from build123d import *

# Parameters (mm, degrees)
SKETCH_1_W            = 40.4
SKETCH_1_H            = 21.6
EXTRUDE_1_DEPTH       = 19.8
SKETCH_3_W            = 38.4
SKETCH_3_H            = 17.9
EXTRUDE_2_DEPTH       = 1
SKETCH_4_W            = 40.4
SKETCH_4_H            = 19.8
EXTRUDE_3_DEPTH       = 0.5
SKETCH_5_R            = 2.75
EXTRUDE_4_DEPTH       = 0.5
EXTRUDE_5_DEPTH       = 0.8
SKETCH_7_R            = 3
EXTRUDE_6_DEPTH       = 2.1
SKETCH_8_R            = 1.9
CUT_EXTRUDE_7_DEPTH   = 38.750231787
SKETCH_10_R           = 0.75
CUT_EXTRUDE_10_DEPTH  = 2.7
EXTRUDE_11_DEPTH      = 1.3
SKETCH_13_R           = 3
CUT_EXTRUDE_13_DEPTH  = 37.710216562
EXTRUDE_START         = -1.3
EXTRUDE_14_DEPTH      = 4.6
SKETCH_14_R           = 2
CUT_EXTRUDE_15_DEPTH  = 39.896915045
EXTRUDE_16_DEPTH      = 0.5
EXTRUDE_16_DEPTH_BACK = 2
SKETCH_15_R           = 2
SKETCH_16_R           = 0.75
CUT_EXTRUDE_17_DEPTH  = 2.3
SKETCH_17_W           = 38.6
SKETCH_17_H           = 18
CUT_EXTRUDE_18_DEPTH  = 20
EXTRUDE_START_2       = 18
SKETCH_18_W           = 38.6
SKETCH_18_H           = 18
EXTRUDE_19_DEPTH      = 18
SKETCH_19_R           = 0.8
CUT_EXTRUDE_20_DEPTH  = 27.4
SKETCH_20_R           = 8.6
CUT_EXTRUDE_21_DEPTH  = 27.4
SKETCH_21_R           = 1.05
EXTRUDE_22_DEPTH      = 0.5
SKETCH_22_R           = 0.75
CUT_EXTRUDE_23_DEPTH  = 0.1
CUT_EXTRUDE_24_REACH  = 37.896
SKETCH_23_R           = 0.5
CUT_EXTRUDE_27_REACH  = 49.887
SKETCH_25_R           = 2
SKETCH_25_W           = 5
SKETCH_25_H           = 1


with BuildPart() as part:
    # 草圖1 → 伸長1 (new body)
    with BuildSketch(Plane.XY):
        Rectangle(SKETCH_1_W, SKETCH_1_H)
    extrude(amount=EXTRUDE_1_DEPTH)

    # 草圖3 → 伸長2 (add)
    with BuildSketch(Plane(origin=(0, 10.8, 0), x_dir=(1, 0, 0), z_dir=(0, 1, 0))):
        with Locations((0, -9.9)):
            Rectangle(SKETCH_3_W, SKETCH_3_H)
        with BuildLine():
            Line((-15.485164876, -1.75), (15.485164876, -1.75))
            ThreePointArc((15.485164876, -1.75), (16.512994231, -3.637005769), (18.4, -4.664835124))
            Line((18.4, -4.664835124), (18.4, -15.135164876))
            ThreePointArc((18.4, -15.135164876), (16.512994231, -16.162994231), (15.485164876, -18.05))
            Line((15.485164876, -18.05), (-15.485164876, -18.05))
            ThreePointArc((-15.485164876, -18.05), (-16.512994231, -16.162994231), (-18.4, -15.135164876))
            Line((-18.4, -15.135164876), (-18.4, -4.664835124))
            ThreePointArc((-18.4, -4.664835124), (-16.512994231, -3.637005769), (-15.485164876, -1.75))
        make_face(mode=Mode.SUBTRACT)
    extrude(amount=EXTRUDE_2_DEPTH)

    # 草圖4 → 伸長3 (add)
    with BuildSketch(Plane(origin=(0, 10.8, 0), x_dir=(1, 0, 0), z_dir=(0, 1, 0))):
        with Locations((0, -9.9)):
            Rectangle(SKETCH_4_W, SKETCH_4_H)
    extrude(amount=EXTRUDE_3_DEPTH)

    # 草圖5 → 伸長4 (add)
    with BuildSketch(Plane(origin=(0, 11.3, 0), x_dir=(1, 0, 0), z_dir=(0, 1, 0))):
        with Locations(Location((-1.55, -9.9, 0), (0, 0, 270))):
            Circle(SKETCH_5_R)
    extrude(amount=EXTRUDE_4_DEPTH)

    # 草圖6 → 伸長5 (add)
    with BuildSketch(Plane(origin=(0, 11.3, 0), x_dir=(1, 0, 0), z_dir=(0, 1, 0))):
        with BuildLine():
            Line((6.2, -7.31930242), (6.2, -12.48069758))
            ThreePointArc((6.2, -12.48069758), (13.6, -9.9), (6.2, -7.31930242))
        make_face()
    extrude(amount=EXTRUDE_5_DEPTH)

    # 草圖7 → 伸長6 (add)
    with BuildSketch(Plane(origin=(0, 12.1, 0), x_dir=(1, 0, 0), z_dir=(0, 1, 0))):
        with Locations(Location((9.45, -9.9, 0), (0, 0, 270))):
            Circle(SKETCH_7_R)
    extrude(amount=EXTRUDE_6_DEPTH)

    # 草圖8 → 伸長7 (cut, through all)
    with BuildSketch(Plane(origin=(0, 14.2, 0), x_dir=(1, 0, 0), z_dir=(0, 1, 0))):
        with Locations(Location((9.45, -9.9, 0), (0, 0, 270))):
            Circle(SKETCH_8_R)
    extrude(amount=-CUT_EXTRUDE_7_DEPTH, mode=Mode.SUBTRACT)

    # 草圖10 → 伸長10 (cut)
    with BuildSketch(Plane(origin=(0, 11.8, 0), x_dir=(1, 0, 0), z_dir=(0, 1, 0))):
        with Locations(Location((-1.55, -9.9, 0), (0, 0, 270))):
            Circle(SKETCH_10_R)
    extrude(amount=-CUT_EXTRUDE_10_DEPTH, mode=Mode.SUBTRACT)

    # 草圖11 → 伸長11 (add)
    with BuildSketch(Plane(origin=(0, 11.3, 0), x_dir=(1, 0, 0), z_dir=(0, 1, 0))):
        with BuildLine():
            Line((-11.95, -5.837980798), (-11.95, -13.962019202))
            ThreePointArc((-11.95, -13.962019202), (-14.95, -9.9), (-11.95, -5.837980798))
        make_face()
    extrude(amount=EXTRUDE_11_DEPTH)

    # 草圖13 → 伸長13 (cut, through all)
    with BuildSketch(Plane(origin=(0, 12.6, 0), x_dir=(1, 0, 0), z_dir=(0, 1, 0))):
        with Locations(Location((-10.7, -9.9, 0), (0, 0, 270))):
            Circle(SKETCH_13_R)
    extrude(amount=-CUT_EXTRUDE_13_DEPTH, mode=Mode.SUBTRACT)

    # 草圖12 → 伸長14 (add)
    with BuildSketch(Plane(origin=(0, 12.6, 0), x_dir=(1, 0, 0), z_dir=(0, 1, 0)).offset(EXTRUDE_START)):
        with BuildLine():
            Line((-9.420351611, -6.75), (-9.420351611, -13.05))
            ThreePointArc((-9.420351611, -13.05), (-14.1, -9.9), (-9.420351611, -6.75))
        make_face()
    extrude(amount=EXTRUDE_14_DEPTH)

    # 草圖14 → 伸長15 (cut, through all)
    with BuildSketch(Plane(origin=(0, 15.9, 0), x_dir=(1, 0, 0), z_dir=(0, 1, 0))):
        with Locations((-10.7, -9.9)):
            Circle(SKETCH_14_R)
    extrude(amount=-CUT_EXTRUDE_15_DEPTH, mode=Mode.SUBTRACT)

    # 草圖15 → 伸長16 (add, two sides: drawn at the far end of the back side and taken through both)
    with BuildSketch(Plane(origin=(0, 15.9, 0), x_dir=(1, 0, 0), z_dir=(0, 1, 0)).offset(-EXTRUDE_16_DEPTH_BACK)):
        with Locations(Location((-10.7, -9.9, 0), (0, 0, 270))):
            Circle(SKETCH_15_R)
    extrude(amount=EXTRUDE_16_DEPTH + EXTRUDE_16_DEPTH_BACK)

    # 草圖16 → 伸長17 (cut)
    with BuildSketch(Plane(origin=(0, 16.4, 0), x_dir=(1, 0, 0), z_dir=(0, 1, 0))):
        with Locations(Location((-10.7, -9.9, 0), (0, 0, 270))):
            Circle(SKETCH_16_R)
    extrude(amount=-CUT_EXTRUDE_17_DEPTH, mode=Mode.SUBTRACT)

    # 草圖17 → 伸長18 (cut)
    with BuildSketch(Plane.XZ.offset(10.8)):
        with Locations((0, 9.9)):
            Rectangle(SKETCH_17_W, SKETCH_17_H)
    extrude(amount=-CUT_EXTRUDE_18_DEPTH, mode=Mode.SUBTRACT)

    # 草圖18 → 伸長19 (add)
    with BuildSketch(Plane.XZ.offset(-9.2).offset(EXTRUDE_START_2)):
        with Locations((0, 9.9)):
            Rectangle(SKETCH_18_W, SKETCH_18_H)
        with BuildLine():
            Line((15.485164876, 1.75), (-15.485164876, 1.75))
            ThreePointArc((-15.485164876, 1.75), (-16.512994231, 3.637005769), (-18.4, 4.664835124))
            Line((-18.4, 4.664835124), (-18.4, 15.135164876))
            ThreePointArc((-18.4, 15.135164876), (-16.512994231, 16.162994231), (-15.485164876, 18.05))
            Line((-15.485164876, 18.05), (15.485164876, 18.05))
            ThreePointArc((15.485164876, 18.05), (16.512994231, 16.162994231), (18.4, 15.135164876))
            Line((18.4, 15.135164876), (18.4, 4.664835124))
            ThreePointArc((18.4, 4.664835124), (16.512994231, 3.637005769), (15.485164876, 1.75))
        make_face(mode=Mode.SUBTRACT)
    extrude(amount=-EXTRUDE_19_DEPTH)

    # 草圖19 → 伸長20 (cut)
    with BuildSketch(Plane(origin=(0, 11.8, 0), x_dir=(1, 0, 0), z_dir=(0, 1, 0))):
        with Locations(Location((-17.7, -2.5, 0), (0, 0, 270))):
            Circle(SKETCH_19_R)
        with Locations(Location((17.7, -2.5, 0), (0, 0, 270))):
            Circle(SKETCH_19_R)
        with Locations(Location((17.7, -17.3, 0), (0, 0, 270))):
            Circle(SKETCH_19_R)
        with Locations(Location((-17.7, -17.3, 0), (0, 0, 270))):
            Circle(SKETCH_19_R)
    extrude(amount=-CUT_EXTRUDE_20_DEPTH, mode=Mode.SUBTRACT)

    # 草圖20 → 伸長21 (cut)
    with BuildSketch(Plane.XZ.offset(-9.2)):
        with Locations((-10.7, 9.9)):
            Circle(SKETCH_20_R)
    extrude(amount=CUT_EXTRUDE_21_DEPTH, mode=Mode.SUBTRACT)

    # 草圖21 → 伸長22 (add)
    with BuildSketch(Plane.XZ.offset(-9.2)):
        with Locations(Location((-1.55, 9.9, 0), (0, 0, 270))):
            Circle(SKETCH_21_R)
    extrude(amount=EXTRUDE_22_DEPTH)

    # 草圖22 → 伸長23 (cut)
    with BuildSketch(Plane(origin=(0, 9.2, 0), x_dir=(1, 0, 0), z_dir=(0, 1, 0))):
        with Locations(Location((-1.55, -9.9, 0), (0, 0, 270))):
            Circle(SKETCH_22_R)
    extrude(amount=-CUT_EXTRUDE_23_DEPTH, mode=Mode.SUBTRACT)

    # 草圖23 → 伸長24 (cut, up to next)
    with BuildSketch(Plane(origin=(0, 11.3, 0), x_dir=(1, 0, 0), z_dir=(0, 1, 0)), mode=Mode.PRIVATE) as cut_extrude_24_sk1:
        with Locations(Location((-10.7, -4.15, 0), (0, 0, 270))):
            Circle(SKETCH_23_R)
    cut_extrude_24_tool1 = extrude(cut_extrude_24_sk1.sketch, amount=-CUT_EXTRUDE_24_REACH, mode=Mode.PRIVATE) & part.part
    # 草圖23 → 伸長24 (cut, up to next)
    with BuildSketch(Plane(origin=(0, 11.3, 0), x_dir=(1, 0, 0), z_dir=(0, 1, 0)), mode=Mode.PRIVATE) as cut_extrude_24_sk2:
        with Locations(Location((-10.7, -15.65, 0), (0, 0, 270))):
            Circle(SKETCH_23_R)
    cut_extrude_24_tool2 = extrude(cut_extrude_24_sk2.sketch, amount=-CUT_EXTRUDE_24_REACH, mode=Mode.PRIVATE) & part.part
    add(cut_extrude_24_tool1.solids().sort_by_distance((-10.7, 11.3, 4.15))[0], mode=Mode.SUBTRACT)
    add(cut_extrude_24_tool2.solids().sort_by_distance((-10.7, 11.3, 15.65))[0], mode=Mode.SUBTRACT)

    # 伸長27: up to this face of the body (flat: up to its plane)
    cut_extrude_27_end = Plane(part.part.faces().sort_by_distance((18.4, 0.2, 9.9))[0])
    # 草圖25 → 伸長27 (cut, up to the picked face)
    with BuildSketch(Plane(origin=(20.2, 0, 0), x_dir=(0, 0, -1), z_dir=(1, 0, 0)), mode=Mode.PRIVATE) as cut_extrude_27_sk1:
        with Locations(Location((-9.9, -3.2, 0), (0, 0, 90))):
            Circle(SKETCH_25_R)
    cut_extrude_27_tool1 = split(extrude(cut_extrude_27_sk1.sketch, amount=-CUT_EXTRUDE_27_REACH, mode=Mode.PRIVATE), bisect_by=cut_extrude_27_end, keep=Keep.BOTH, mode=Mode.PRIVATE)
    # 草圖25 → 伸長27 (cut, up to the picked face)
    with BuildSketch(Plane(origin=(20.2, 0, 0), x_dir=(0, 0, -1), z_dir=(1, 0, 0)), mode=Mode.PRIVATE) as cut_extrude_27_sk2:
        with Locations((-9.9, -10.3)):
            Rectangle(SKETCH_25_W, SKETCH_25_H)
    cut_extrude_27_tool2 = split(extrude(cut_extrude_27_sk2.sketch, amount=-CUT_EXTRUDE_27_REACH, mode=Mode.PRIVATE), bisect_by=cut_extrude_27_end, keep=Keep.BOTH, mode=Mode.PRIVATE)
    add(cut_extrude_27_tool1.solids().sort_by(Axis((20.2, -3.2, 9.9), (-1, 0, 0)))[0], mode=Mode.SUBTRACT)
    add(cut_extrude_27_tool2.solids().sort_by(Axis((20.2, -10.3, 9.9), (-1, 0, 0)))[0], mode=Mode.SUBTRACT)


solid = part.part
For this review, take the finished solid that the model builds, in its own axes (mm). A direction names the side the tool comes from. Give positions to 0.01 mm unless a question says otherwise; leave off trailing zeros. Order: outer loops, then holes, each group sorted by start corner. A loop starts at its lowest first (then second) coordinate and runs counter-clockwise, first axis right, second up. Notation, with made-up numbers: (-36, 81.5) -> (15, 81.5) arc R15 ccw to (15, 109.5) -> close; hole circle Ø1 at (15.25, 32.5). An arc over 180 degrees is marked (long way). Write item = value, one per line.
1) To check wall thickness, follow L1, parallel to Z at x = -10.5, y = 6; L2, parallel to Z at x = -11.5, y = -9.25; L3, parallel to X at y = -9, z = 14.5. State the ranges of each line that lie inside material, in increasing order. Write a range as from..to.
Findings:
L1 = 0..1.3, 18.5..19.8
L2 = 0..0.9, 18.9..19.8
L3 = -20.2..-19.3, 19.3..20.2
2) Insertion check: pin 1 (2.5 mm diameter, centred on x = 17.7, z = 2.5, fed in from -Y); pin 2 (0.6 mm diameter, centred on x = -6.5, y = 11.5, fed in from +Z); pin 3 (6 mm diameter, centred on x = -1.5, z = 8, fed in from +Y); pin 4 (0.6 mm diameter, centred on x = -1, z = 10, fed in from -Y). Each pin has a flat end and moves straight along its axis. Give the tip position at first contact, or say it passes through.
Findings:
pin_1 = -8.8
pin_2 = 19.8
pin_3 = 11.8
pin_4 = 8.7
3) We need section B-B, the plane y = 10.25. Count the separate pieces of the cut face and the enclosed holes in it, and give its area (3 significant figures).
Findings:
separate_pieces = 1
enclosed_holes = 9
area = 749 mm^2
4) We need section C-C, the plane y = 4.75. Give the boundary of the cut face in (x, z).
Findings:
outline = (-20.2, 0) -> (20.2, 0) -> (20.2, 19.8) -> (-20.2, 19.8) -> close; hole circle Ø1.6 at (-17.7, 2.5); hole circle Ø1.6 at (-17.7, 17.3); hole (-18.4, 4.66) arc R3.8 cw to (-17.01, 4.05) arc R8.6 ccw to (-16.21, 3.3) arc R3.8 cw to (-15.49, 1.75) -> (-13.45, 1.75) arc R8.6 ccw to (-7.95, 1.75) -> (15.49, 1.75) arc R3.8 cw to (18.4, 4.66) -> (18.4, 15.14) arc R3.8 cw to (15.49, 18.05) -> (-7.95, 18.05) arc R8.6 ccw to (-13.45, 18.05) -> (-15.49, 18.05) arc R3.8 cw to (-16.21, 16.5) arc R8.6 ccw to (-17.01, 15.75) arc R3.8 cw to (-18.4, 15.14) -> (-18.4, 13.73) arc R8.6 ccw to (-18.4, 6.07) -> close; hole circle Ø1.6 at (17.7, 2.5); hole circle Ø1.6 at (17.7, 17.3)
5) For faces 1 (the face through (-18.4, 0, 5)), 2 (the face through (6.2, 11.7, 9.9)), 3 (the face through (-2, 11.8, 9)), list the 3-axis set-ups (+Z, -Z, +X, -X, +Y, -Y) from which the entire face can be reached by the end or side of a thin tool; tool diameter is ignored.
Findings:
face_1 = -Y
face_2 = +Y
face_3 = +Z, -Z, +Y
6) Draft analysis for pull direction Z (two halves, no side actions). For faces 4 (the face through (19.313, -2.277, 8.126)), 5 (the face through (-12, 16.4, 10)), 6 (the face through (0, 0, 19.8)), state which applies: pulls with the +Z half, pulls with the -Z half, needs draft (parallel to the pull), parting line crosses it, or undercut.
Findings:
face_4 = undercut
face_5 = needs draft
face_6 = pulls with the +Z half
7) We need section D-D, the plane z = 17.3. Give the boundary of the cut face in (x, y), and give its area (3 significant figures).
Findings:
outline = (-20.2, -10.8) -> (-19.3, -10.8) -> (-19.3, -8.8) -> (-18.5, -8.8) -> (-18.5, 11.8) -> (-19.2, 11.8) -> (-19.2, 11.3) -> (-20.2, 11.3) -> close; (-16.9, -8.8) -> (-15.73, -8.8) -> (-15.73, 9.2) -> (15.73, 9.2) -> (15.73, -8.8) -> (16.9, -8.8) -> (16.9, 11.8) -> (15.73, 11.8) -> (15.73, 11.3) -> (-15.73, 11.3) -> (-15.73, 11.8) -> (-16.9, 11.8) -> close; (18.5, -8.8) -> (19.3, -8.8) -> (19.3, -10.8) -> (20.2, -10.8) -> (20.2, 11.3) -> (19.2, 11.3) -> (19.2, 11.8) -> (18.5, 11.8) -> close
area = 187 mm^2
